Geometry check sheet. Reference: the model listing, model coordinates, mm. Face numbers are marked on the shaded views. A direction names the side the tool comes from. Give positions to 0.01 mm unless a question says otherwise; leave off trailing zeros. Loops run counter-clockwise (first coordinate to the right, second up) from the corner with the lowest first, then second, coordinate; pieces in that order, holes last.
1. Cross-section at B-B, the plane x = -17. Record the cut outline in (y, z).
2. Release check for a two-part mould opening along Z. For the marked faces 1, 2, 3 and 4 record: +Z half, -Z half, draft (parallel to the pull), parting line (faces both ways), or undercut.
3. Cross-section at C-C, the plane z = 14.75. Record the cut outline in (x, y), plus the area to 3 significant figures.
4. Material ranges on L1, parallel to Z at x = 0, y = -1.75; L2, parallel to X at y = 0, z = 2.1; L3, parallel to Z at x = 0, y = 0.75, recorded low to high.
5. Go/stop test with flat-tipped pins: pin 1 Ø3 at (x, z) = (-0.5, 13) entering from +Y; pin 2 Ø2 at (x, z) = (-8.75, 5) entering from +Y; pin 3 Ø3.5 at (x, y) = (-17, 0) entering from -Z. Record where each tip stops, or that it passes through.
6. Tool access check on the marked faces 5 and 6. Record the directions out of +Z, -Z, +X, -X, +Y, -Y that give a thin tool (end or side, any length) a straight path to the whole face; none if there is none.
7. Cross-section at D-D, the plane z = 2.75. Record the cut outline in (x, y), plus the area to 3 significant figures.
8. Cross-section at A-A, the plane y = 0. State how many separate pieces and enclosed holes the cut face has, plus the area to 3 significant figures.
Solid Edge part; units mm, degrees
sketch "Sketch1" plane through (0, 0, 0) normal (0, -1, 0) x (1, 0, 0)
  line L0 (-20, 5) -> (-20, 0)
  line L1 (-20, 0) -> (20, 0)
  line L2 (20, 0) -> (20, 5)
  line L3 (20, 5) -> (14, 5)
  line L4 (14, 5) -> (10, 20)
  line L5 (10, 20) -> (-10, 20)
  line L6 (-10, 20) -> (-14, 5)
  line L7 (-14, 5) -> (-20, 5)
  dimension "D1" = 10
  dimension "D2" = 20
  dimension "D3" = 20
  dimension "D4" = 14
extrude "Protrusion1" add sketch "Sketch1" along normal mid plane 6
fillet "rounds" radius 3 2 edges at (10, 0, 20) (-10, 0, 20)
hole "Hole1" at (0, 3, 13.75) direction (0, -1, 0) diameter 3.4 end up to next counterbore diameter 6.5 counterbore depth 3.5
hole "Hole2" at (8.75, 3, 5) direction (0, -1, 0) diameter 3.4 end up to next counterbore diameter 6.5 counterbore depth 3.5
hole "Hole3" at (-8.75, 3, 5) direction (0, -1, 0) diameter 3.4 end up to next counterbore diameter 6.5 counterbore depth 3.5
hole "Hole4" at (-17, 0, 5) direction (0, 0, -1) diameter 3.2 end up to next start chamfer 0.3 start chamfer angle 45 end chamfer 0.3 end chamfer angle 45
hole "Hole5" at (17, 0, 5) direction (0, 0, -1) diameter 3.2 end up to next start chamfer 0.3 start chamfer angle 45 end chamfer 0.3 end chamfer angle 45
properties material "Polyethylene, low density"
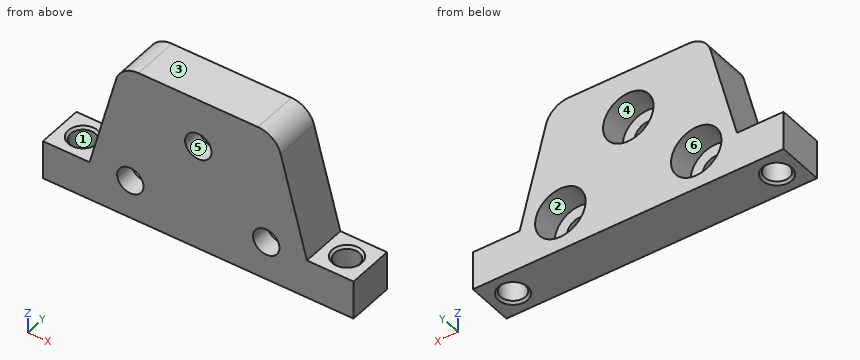
Result:
1. outline: (-3, 0) - (-1.9, 0) - (-1.6, 0.3) - (-1.6, 4.7) - (-1.9, 5) - (-3, 5) - close; (1.6, 0.3) - (1.9, 0) - (3, 0) - (3, 5) - (1.9, 5) - (1.6, 4.7) - close
2. face 1: draft
2. face 2: undercut
2. face 3: +Z half
2. face 4: undercut
3. outline: (-11.4, -3) - (-1.37, -3) - (-1.37, -0.5) - (-3.09, -0.5) - (-3.09, 3) - (-11.4, 3) - close; (1.37, -3) - (11.4, -3) - (11.4, 3) - (3.09, 3) - (3.09, -0.5) - (1.37, -0.5) - close
3. area: 108 mm2
4. L1: z = 0 to 12.05, 15.45 to 20
4. L2: x = -20 to -18.6, -15.4 to -10.22, -7.28 to 7.28, 10.22 to 15.4, 18.6 to 20
4. L3: z = 0 to 10.5, 17 to 20
5. pin 1: stops at y = -0.5
5. pin 2: passes through
5. pin 3: stops at z = 0.15
6. face 5: +Y, -Y
6. face 6: +Y
7. outline: (-20, -3) - (20, -3) - (20, 3) - (11.1, 3) - (11.1, -0.5) - (6.4, -0.5) - (6.4, 3) - (-6.4, 3) - (-6.4, -0.5) - (-11.1, -0.5) - (-11.1, 3) - (-20, 3) - close; hole circle Ø3.2 at (-17, 0); hole circle Ø3.2 at (17, 0)
7. area: 191 mm2
8. separate pieces: 3
8. enclosed holes: 3
8. area: 426 mm2
